Geometry: final body of the model. Coordinates: model frame, mm. A direction names the side the tool comes from. Round coordinates to 2 decimals unless told otherwise and drop trailing zeros. Loops run counter-clockwise (first coordinate to the right, second up) from the corner with the lowest first, then second, coordinate; pieces in that order, holes last. Notation, with made-up numbers: (-21, 6) - (23, 6) arc R22 cw to (23, 25) - close; hole circle Ø10 at (-9, -32.75). An arc over 180 degrees is marked (long way). Answer as a JSON object with one key per item and string values. Group by question number.
Item 1: Reachability of faces 1 (the face through (-25, 10, -11)), 2 (the face through (-10.1, 8.5, 17)), 3 (the face through (-13, 3, 15)) from +Z, -Z, +X, -X, +Y, -Y: full face, straight path, thin tool, end or side. Return the list, or none.
Item 2: Section D-D (x = 9). Count the separate pieces of the cut face and the enclosed holes in it, plus the area to 3 significant figures.
Item 3: Section B-B (x = -6.5). Return the cut outline in (y, z).
Item 4: First-contact query: pin 1 (5 mm diameter, centred on y = 12, z = 16, fed in from -X); pin 2 (3 mm diameter, centred on y = 9.5, z = 17, fed in from +X); pin 3 (1.5 mm diameter, centred on y = 16, z = -6.5, fed in from -X); pin 4 (16 mm diameter, centred on x = 0, z = 0, fed in from -Y). Flat tips, straight axial feed; report the tip coordinate or a pass-through.
Item 5: Section A-A (y = 10). Return the cut outline in (x, z), plus the area to 3 significant figures.
Item 6: Section C-C (x = -23). Return the cut outline in (y, z).
Item 7: Line query: line 1 (X direction, y = 15.5, z = 0); line 2 (Y direction, x = 7, z = 15); line 3 (X direction, y = 1.25, z = 1.5). Output: solid intervals per line, ascending.
Item 8: Draft query along X for faces 4 (the face through (-13, 10, 20)), 5 (the face through (11, 8, 13)), 6 (the face through (-0.5, 10, 12)). Return one class per face: released by +X, released by -X, zero draft, split by the parting line, or undercut.
```python
from build123d import *
from build123d.topology import SkipClean

# Parameters (mm, degrees)
BOSS_EXTRUDE1_DEPTH = 20
SKETCH2_R           = 5
BOSS_EXTRUDE2_DEPTH = 41
CUT_EXTRUDE1_DEPTH  = 41
SKETCH4_R           = 2.5
CUT_EXTRUDE2_DEPTH  = 31
FILLET1_R           = 2
SKETCH5_R           = 10
BOSS_EXTRUDE3_DEPTH = 15
CUT_EXTRUDE3_DEPTH  = 5
CHAMFER1_SIZE       = 2


with BuildPart() as part:
    # Sketch1 → Boss-Extrude1 (new body)
    with BuildSketch(Plane(origin=(0, 0, 0), x_dir=(1, 0, 0), z_dir=(0, 1, 0))):
        with BuildLine():
            ThreePointArc((0.5, -14.991664351), (14.997915943, 0.250034739), (0, 15))
            Line((0, 15), (-30, 15))
            Line((-30, 15), (-30, -15))
            Line((-30, -15), (-0.5, -15))
            Line((-0.5, -15), (-0.5, -9.987492178))
            ThreePointArc((-0.5, -9.987492178), (0, 10), (0.5, -9.987492178))
            Line((0.5, -9.987492178), (0.5, -14.991664351))
        make_face()
    extrude(amount=BOSS_EXTRUDE1_DEPTH)

    # Sketch2 → Boss-Extrude2 (add)
    with BuildSketch(Plane.ZY.offset(30)):
        with Locations(Location((15, 10, 0), (0, 0, 270))):
            Circle(SKETCH2_R)
    extrude(amount=-BOSS_EXTRUDE2_DEPTH)

    # Sketch3 → Cut-Extrude1 (cut)
    with BuildSketch(Plane(origin=(0, 20, 0), x_dir=(1, 0, 0), z_dir=(0, 1, 0))):
        Polygon((-0.5, -15), (-0.5, -9.987492178), (0.5, -9.987492178), (0.5, -14.991664351), (0.5, -20), (-0.5, -20), align=None)
    extrude(amount=-CUT_EXTRUDE1_DEPTH, mode=Mode.SUBTRACT)

    # Sketch4 → Cut-Extrude2 (cut)
    with BuildSketch(Plane(origin=(11, 0, 0), x_dir=(0, 0, -1), z_dir=(1, 0, 0))):
        with Locations((-15, 10)):
            Circle(SKETCH4_R)
    extrude(amount=-CUT_EXTRUDE2_DEPTH, mode=Mode.SUBTRACT)

    # Fillet1
    fillet1_edges = [part.edges().sort_by_distance(p)[0] for p in [
        (-15, 0, -15),
        (14.997915943, 0, -0.250034739),
        (-15, 20, -15),
        (-15.25, 20, 15),
        (14.997915943, 20, -0.250034739),
        (-15.25, 0, 15),
    ]]
    fillet(fillet1_edges, radius=FILLET1_R)

    # Sketch5 → Boss-Extrude3 (add)
    with BuildSketch(Plane.ZY.offset(30)):
        with Locations(Location((0, 10, 0), (0, 0, 270))):
            Circle(SKETCH5_R)
    extrude(amount=BOSS_EXTRUDE3_DEPTH)

    # Sketch6 → Cut-Extrude3 (cut)
    with SkipClean():  # the faces are left unmerged after this step: merging them gives an invalid solid
        with BuildSketch(Plane.ZY.offset(30)):
            with BuildLine():
                ThreePointArc((0, 0), (-10, 10), (0, 20))
                Line((0, 20), (-13, 20))
                ThreePointArc((-13, 20), (-14.414213562, 19.414213562), (-15, 18))
                Line((-15, 18), (-15, 2))
                ThreePointArc((-15, 2), (-14.414213562, 0.585786438), (-13, 0))
                Line((-13, 0), (0, 0))
            make_face()
            with BuildLine():
                Line((13, 20), (0, 20))
                ThreePointArc((0, 20), (10, 10), (0, 0))
                Line((0, 0), (13, 0))
                ThreePointArc((13, 0), (14.414213562, 0.585786438), (15, 2))
                Line((15, 2), (15, 5))
                ThreePointArc((15, 5), (20, 10), (15, 15))
                Line((15, 15), (15, 18))
                ThreePointArc((15, 18), (14.414213562, 19.414213562), (13, 20))
            make_face()
        extrude(amount=-CUT_EXTRUDE3_DEPTH, mode=Mode.SUBTRACT)

    # Chamfer1
    chamfer1_edges = [part.edges().sort_by_distance(p)[0] for p in [
        (-45, 20, 0),
    ]]
    chamfer(chamfer1_edges, length=CHAMFER1_SIZE)


solid = part.part
```
Values:
{
 "1": {"face 1": "-Z, -X", "face 2": "+X", "face 3": "+Z, +X, -X, -Y"},
 "2": {"separate pieces": "2", "enclosed holes": "1", "area": "349 mm^2"},
 "3": {"outline": "(0, -13) arc R2 ccw to (2, -15) - (18, -15) arc R2 ccw to (20, -13) - (20, -7.6) - (0, -7.6) - close; (0, 7.6) - (20, 7.6) - (20, 13) arc R2 ccw to (18, 15) - (15, 15) arc R5 ccw to (5, 15) - (2, 15) arc R2 ccw to (0, 13) - close; hole circle Ø5 at (10, 15)"},
 "4": {"pin 1": "stops at x = -25", "pin 2": "stops at x = 11", "pin 3": "stops at x = -44.9", "pin 4": "passes through"},
 "5": {"outline": "(-45, -8) - (-43, -10) - (-25, -10) - (-25, -15) - (0, -15) arc R15 ccw to (11, 10.2) - (11, 12.5) - (0.5, 12.5) - (0.5, 9.99) arc R10 cw (long way) to (-0.5, 9.99) - (-0.5, 12.5) - (-20, 12.5) - (-20, 17.5) - (-0.5, 17.5) - (-0.5, 20) - (-25, 20) - (-25, 10) - (-43, 10) - (-45, 8) - close; (0.5, 17.5) - (11, 17.5) - (11, 20) - (0.5, 20) - close", "area": "1,220 mm^2"},
 "6": {"outline": "(0, -13) arc R2 ccw to (2, -15) - (18, -15) arc R2 ccw to (20, -13) - (20, 13) arc R2 ccw to (18, 15) - (15, 15) arc R5 ccw to (5, 15) - (2, 15) arc R2 ccw to (0, 13) - close"},
 "7": {"line 1": "x = -45 to -10, 10 to 15", "line 2": "y = 5 to 7.5, 12.5 to 15", "line 3": "x = -44.12 to -9.89, 9.89 to 14.78"},
 "8": {"face 4": "zero draft", "face 5": "released by +X", "face 6": "undercut"}
}
